Part model, mm, in its own coordinate system. A direction names the side the tool comes from. Give positions to 0.01 mm unless a question says otherwise; leave off trailing zeros. Write each loop counter-clockwise with the first axis right and the second up, starting at its lowest first coordinate (ties: lowest second). Pieces come first, ordered by that corner, then holes. Notation, with made-up numbers: (47, 83) - (80, 83) arc R21 ccw to (80, 116) - close; hole circle Ø1 at (-13, 42.25). An arc over 180 degrees is marked (long way). Answer as a JSON object with one key per item and string values. Group by question number.
```python
from build123d import *

# Parameters (mm, degrees)
F0_R     = 40.65
F0_R_2   = 34.15
F1_DEPTH = 2
F2_R     = 40.65
F2_R_2   = 40
F3_DEPTH = 3
F4_R     = 34.65
F4_R_2   = 34.15
F5_DEPTH = 3
F6_R     = 1.25
F7_DEPTH = 25


with BuildPart() as f1:
    # F0 (on Front) → F1 (new body)
    with BuildSketch(Plane.XZ):
        Circle(F0_R)
        Circle(F0_R_2, mode=Mode.SUBTRACT)
    extrude(amount=F1_DEPTH)

    # F2 (on face) → F3 (join)
    with BuildSketch(Plane.XZ.offset(2)):
        Circle(F2_R)
        Circle(F2_R_2, mode=Mode.SUBTRACT)
    extrude(amount=F3_DEPTH)

    # F4 (on face) → F5 (join)
    with BuildSketch(Plane.XZ.offset(2)):
        Circle(F4_R)
        Circle(F4_R_2, mode=Mode.SUBTRACT)
    extrude(amount=F5_DEPTH)

    # F6 (on face) → F7 (cut)
    with BuildSketch(Plane.XZ.offset(2)):
        with Locations((1.767338, 37.755713)):
            Circle(F6_R)
    extrude(amount=-F7_DEPTH, mode=Mode.SUBTRACT)


solid = f1.part
```
1) Saw through at C-C (x = -14). List the corners of the cut face in (y, z), and give its area (3 significant figures).
2) Drill centre lines: line 1 along Z through (x, y) = (0, -2.5); line 2 along Z through (x, y) = (31.5, -2.75); line 3 along X through (y, z) = (-2.4, -6.5). Where is each one in solid material? Low to high. Write a range as from..to.
3) Which spindle directions (+Z, -Z, +X, -X, +Y, -Y) get a long thin tool onto all of the face, cutting with end or side? Do faces 4 (the cylindrical face through (33.05, -3.48, 10.41)), 5 (the cylindrical face through (-7.4, -2.46, -33.34)). Say none if no direction does.
4) Saw through at A-A (z = 0). List the corners of the cut face in (x, y), and give its area (3 significant figures).
5) Two-plate mould, pull along X, no slides. Class faces 1 (the cylindrical face through (2.344, -1.014, 36.647)), 2 (the cylindrical face through (38.773, -2.465, 12.21)), 3 (the flat face through (30, -5, -27)): +X half, -X half, draft (parallel to the pull), parting line (faces both ways), or undercut.
6) Saw through at B-B (y = -2.75). List the corners of the cut face in (x, z).
7) Drop flat-ended pins along their axis: P1, Ø2, axis at x = 11, y = -1, coming from the -Z side; P2, Ø3, axis at y = -1, z = -6.5, coming from the +X side; P3, Ø5, axis at x = -32, z = 24.5, coming from the +Y side; P4, Ø3, axis at x = 1.77, z = 37.76, coming from the -Y side. Give the stop position or say it passes through.
Checks:
{
 "1": {"outline": "(-5, -38.16) - (0, -38.16) - (0, -31.15) - (-5, -31.15) - (-5, -31.7) - (-2, -31.7) - (-2, -37.47) - (-5, -37.47) - close; (-5, 31.15) - (0, 31.15) - (0, 38.16) - (-5, 38.16) - (-5, 37.47) - (-2, 37.47) - (-2, 31.7) - (-5, 31.7) - close", "area": "35.5 mm2"},
 "2": {"line 1": "-40.65..-40, -34.65..-34.15, 34.15..34.65, 40..40.65", "line 2": "-25.69..-24.65, -14.44..-13.19, 13.19..14.44, 24.65..25.69", "line 3": "-40.13..-39.47, -34.03..-33.53, 33.53..34.03, 39.47..40.13"},
 "3": {"face 4": "-Y", "face 5": "+Y, -Y"},
 "4": {"outline": "(-40.65, -5) - (-40, -5) - (-40, -2) - (-34.65, -2) - (-34.65, -5) - (-34.15, -5) - (-34.15, 0) - (-40.65, 0) - close; (34.15, -5) - (34.65, -5) - (34.65, -2) - (40, -2) - (40, -5) - (40.65, -5) - (40.65, 0) - (34.15, 0) - close", "area": "32.9 mm2"},
 "5": {"face 1": "undercut", "face 2": "parting line", "face 3": "draft"},
 "6": {"outline": "circle Ø81.3 at (0, 0); circle Ø69.3 at (0, 0); hole circle Ø80 at (0, 0); hole circle Ø68.3 at (0, 0)"},
 "7": {"P1": "z = -39.4", "P2": "x = 40.34", "P3": "y = 0", "P4": "y = -2"}
}
